Build history of the part. All positions in model axes, mm. Face numbers are marked on the shaded views. A direction names the side the tool comes from. Coordinates: 2 decimals unless noted, no trailing zeros. Write each loop counter-clockwise with the first axis right and the second up, starting at its lowest first coordinate (ties: lowest second). Pieces come first, ordered by that corner, then holes.
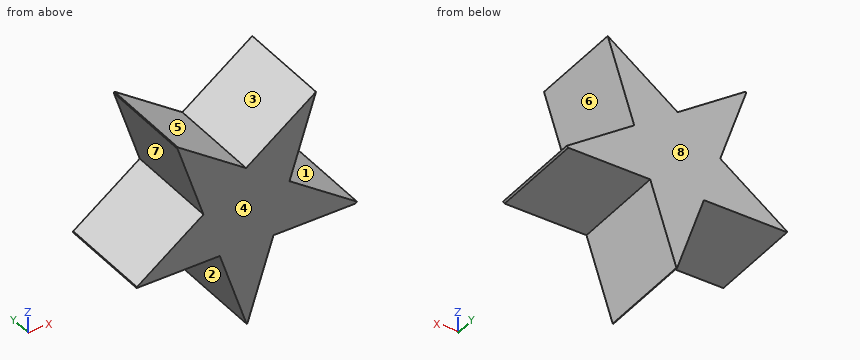
```python
from build123d import *

# Parameters (mm, degrees)
F2_DEPTH = 38.1


with BuildPart() as f2:
    # F1 (on face) → F2 (new body)
    with BuildSketch(Plane.XZ):
        Polygon((0.1359417947, -47.3937628545), (10.7827526257, -14.8319200301), (-11.0337428161, -14.4123720925), (-0.1378061081, -47.3924083515), (0, -47.4925303496), align=None)
        Polygon((44.7767423867, -14.9603227402), (17.2892784216, 5.0674163686), (10.7827526257, -14.8319200301), (44.0723355844, -15.472104239), align=None)
        Polygon((-17.6862078163, 5.7234402568), (-0.3723328356, 17.935905908), (-28.025253062, 38.0841986931), (-28.1999326712, 37.5465901356), align=None)
        Polygon((-11.0337428161, -14.4123720925), (-17.6862078163, 5.7234402568), (-44.7402710109, -13.3593368718), (-44.8709923662, -13.7616558351), align=None)
        Polygon((17.2892784216, 5.0674163686), (28.0526187271, 37.9856489599), (-0.3723328356, 17.935905908), align=None)
        Polygon((10.7827526257, -14.8319200301), (17.2892784216, 5.0674163686), (-0.3723328356, 17.935905908), (-17.6862078163, 5.7234402568), (-11.0337428161, -14.4123720925), align=None)
    extrude(amount=F2_DEPTH)


solid = f2.part
```
1. Probe line 1 along X through (y, z) = (-8, 19.5); line 2 along Z through (x, y) = (-36, -31); line 3 along Z through (x, y) = (-15.5, -2). List the from-to ranges inside material, lowest first.
Computed values:
line 1: x = -22.24 to -2.52, 1.85 to 22.01
line 2: z = -13.93 to -7.19
line 3: z = -14.33 to 28.96
2. Flat gauge pins, fed straight in: pin 1 (1 mm diameter, centred on x = -34.5, y = -23.5, fed in from -Z); pin 2 (6 mm diameter, centred on y = -30, z = 18, fed in from -X); pin 3 (12 mm diameter, centred on y = -24, z = 24.5, fed in from -X). Where does each tip first touch, or does it go through?
Computed values:
pin 1: stops at z = -13.97
pin 2: stops at x = -22.73
pin 3: stops at x = -25.87
3. Saw through at D-D on z = -32.5. List the corners of the cut face in (x, y), plus the area to 3 significant figures.
Computed values:
outline: (-5.06, -38.1) - (5.01, -38.1) - (5.01, 0) - (-5.06, 0) - close
area: 383 mm2
4. Saw through at C-C on y = -32.5. List the corners of the cut face in (x, z).
Computed values:
outline: (-44.87, -13.76) - (-11.03, -14.41) - (-0.14, -47.39) - (0, -47.49) - (0.14, -47.39) - (10.78, -14.83) - (44.07, -15.47) - (44.78, -14.96) - (17.29, 5.07) - (28.05, 37.99) - (-0.37, 17.94) - (-28.03, 38.08) - (-28.2, 37.55) - (-17.69, 5.72) - (-44.74, -13.36) - close
5. 3-axis set-ups, long thin cutter, end or side, ignore diameter. For the marked faces 4, 5, 6, 7 and 8: which of +Z, -Z, +X, -X, +Y, -Y reach the whole face in a straight line?
Computed values:
face 4: +Z, -Z, +X, -X, -Y
face 5: +Z, +Y, -Y
face 6: +X, +Y, -Y
face 7: -X, +Y, -Y
face 8: +Z, -Z, +X, -X, +Y
6. Mould opens along X. For the marked faces 1, 2 and 3 say: +X half, -X half, draft (parallel to the pull), parting line (faces both ways), or undercut.
Computed values:
face 1: +X half
face 2: -X half
face 3: undercut
7. Saw through at A-A on z = 29. List the corners of the cut face in (x, y).
Computed values:
outline: (-25.38, -38.1) - (-15.56, -38.1) - (-15.56, 0) - (-25.38, 0) - close; (15.31, -38.1) - (25.11, -38.1) - (25.11, 0) - (15.31, 0) - close
8. Saw through at B-B on x = -19.5. List the corners of the cut face in (y, z), plus the area to 3 significant figures.
Computed values:
outline: (-38.1, -14.25) - (0, -14.25) - (0, 4.44) - (-38.1, 4.44) - close; (-38.1, 11.21) - (0, 11.21) - (0, 31.87) - (-38.1, 31.87) - close
area: 1,500 mm2
